Part model, mm, in its own coordinate system. Face numbers are marked on the shaded views. A direction names the side the tool comes from. Give positions to 0.01 mm unless a question says otherwise; leave off trailing zeros. Write each loop counter-clockwise with the first axis right and the second up, starting at its lowest first coordinate (ties: lowest second). Pieces come first, ordered by that corner, then holes. Notation, with made-up numbers: M -5.5,-8 L 44.5,-8 A23 ccw 44.5,16 Z; hole C 49,21 d2. An arc over 180 degrees is marked long. Answer as CSV lines item,"result". Start each with the question number.
Item 1: Pin check, flat tips, straight feed: pin 1 (8 mm diameter, centred on x = 12, y = -66.5, fed in from +Z); pin 2 (10.5 mm diameter, centred on x = -5, y = 8.5, fed in from -Z); pin 3 (3 mm diameter, centred on x = -12.5, z = -0.5, fed in from +Y); pin 4 (5 mm diameter, centred on y = -50, z = -5, fed in from -X). Stop position of each tip, or through.
Item 2: Band-saw the part on B-B, the plane z = 0. List the corners of the cut face in (x, y) (3 decimals), then the cut area to 3 significant figures.
Item 3: Band-saw the part on A-A, the plane x = 0. List the corners of the cut face in (y, z) (3 decimals), then the cut area to 3 significant figures.
Item 4: Band-saw the part on D-D, the plane y = -73. List the corners of the cut face in (x, z) (3 decimals), then the cut area to 3 significant figures.
Item 5: Band-saw the part on C-C, the plane y = 0. List the corners of the cut face in (x, z) (3 decimals).
Item 6: Wall check: L1, parallel to Y at x = 0.5, z = -96; L2, parallel to Y at x = 3.5, z = -101; L3, parallel to X at y = 51, z = -4. Give the ranges that are in metal, low to high. Write a range as from..to.
Item 7: 3-axis set-ups, long thin cutter, end or side, ignore diameter. For the marked faces 1 and 2: which of +Z, -Z, +X, -X, +Y, -Y reach the whole face in a straight line?
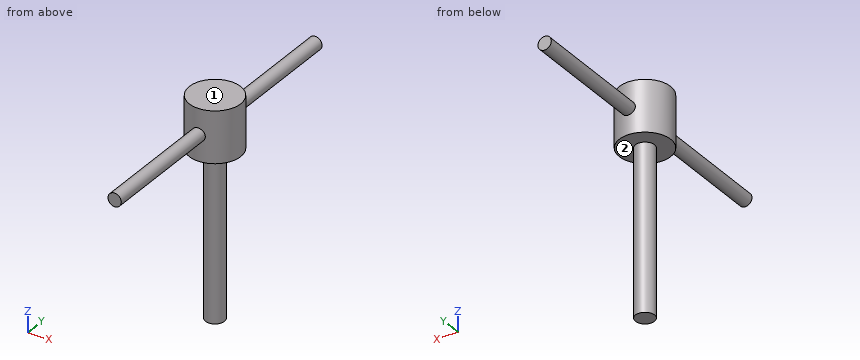
from build123d import *

# Parameters (mm, degrees)
F0_R          = 17.145
F1_DEPTH      = 17.145
F2_W          = 6.35
F2_H          = 110.54443
F4_R          = 4.445
F5_DEPTH      = 17.146
F5_DEPTH_BACK = 25.4
F6_R          = 4.445
F7_DEPTH      = 101.6


with BuildPart() as f1:
    # F0 (on Top) → F1 (new body, symmetric)
    with BuildSketch(Plane.XY):
        Circle(F0_R)
    extrude(amount=F1_DEPTH, both=True)

    # F2 (on Front) → F3 (revolve)
    with BuildSketch(Plane.XZ):
        with Locations((-3.175, -72.417215)):
            Rectangle(F2_W, F2_H)
    revolve(axis=Axis((0, 0, -76.082058), (0, 0, -1)))

    # F4 (on Front) → F5 (cut, two sides)
    with BuildSketch(Plane.XZ) as f5_sk:
        Circle(F4_R)
    extrude(amount=-F5_DEPTH, mode=Mode.SUBTRACT)
    extrude(f5_sk.sketch, amount=-F5_DEPTH_BACK, mode=Mode.SUBTRACT)

    # F6 (on Front) → F7 (join, symmetric)
    with BuildSketch(Plane.XZ):
        Circle(F6_R)
    extrude(amount=F7_DEPTH, both=True)


solid = f1.part
Output:
1,pin 1,"through"
1,pin 2,"z = -127.69"
1,pin 3,"y = 13.15"
1,pin 4,"x = -3.68"
2,outline,"M -4.445,-101.6 L 4.445,-101.6 L 4.445,-16.559 A17.145 ccw 4.445,16.559 L 4.445,101.6 L -4.445,101.6 L -4.445,16.559 A17.145 ccw -4.445,-16.559 Z"
2,area,"2,430 mm²"
3,outline,"M -101.6,-4.445 L -17.145,-4.445 L -17.145,-17.145 L -6.35,-17.145 L -6.35,-127.689 L 6.35,-127.689 L 6.35,-17.145 L 17.145,-17.145 L 17.145,-4.445 L 101.6,-4.445 L 101.6,4.445 L 17.145,4.445 L 17.145,17.145 L -17.145,17.145 L -17.145,4.445 L -101.6,4.445 Z"
3,area,"4,080 mm²"
4,outline,"C 0,0 d8.89"
4,area,"62.1 mm²"
5,outline,"M -17.145,-17.145 L -6.35,-17.145 L -6.35,-127.689 L 6.35,-127.689 L 6.35,-17.145 L 17.145,-17.145 L 17.145,17.145 L -17.145,17.145 Z"
6,L1,"-6.33..6.33"
6,L2,"-5.3..5.3"
6,L3,"-1.94..1.94"
7,face 1,"+Z, +X, -X, +Y, -Y"
7,face 2,"-Z"
